For this review, take the finished solid that the model builds, in its own axes (mm). A direction names the side the tool comes from. Round coordinates to 2 decimals unless told otherwise and drop trailing zeros. Write each loop counter-clockwise with the first axis right and the second up, starting at its lowest first coordinate (ties: lowest second). Pieces come first, ordered by that corner, then holes. Notation, with made-up numbers: (88, 82) - (118, 82) arc R9 ccw to (118, 86) - close; hole circle Ø10 at (63.25, -40). An arc over 180 degrees is marked (long way). Answer in a Markdown table with one row per item. Add a question column.
from build123d import *

# Parameters (mm, degrees)
SKETCH1_R                 = 21
BOSS_EXTRUDE1_DEPTH       = 2
SKETCH2_R                 = 20
BOSS_EXTRUDE2_DEPTH       = 74
SKETCH3_R                 = 12.5
CUT_EXTRUDE1_DEPTH        = 77
SKETCH4_W                 = 8
SKETCH4_H                 = 7
CUT_EXTRUDE2_DEPTH        = 76
M6X1_0_TAPPED_HOLE1_D     = 5
M6X1_0_TAPPED_HOLE1_DEPTH = 8.497848452
M6X1_0_TAPPED_HOLE1_TIP   = 1.502151548


with BuildPart() as part:
    # Sketch1 → Boss-Extrude1 (new body)
    with BuildSketch(Plane.XY):
        Circle(SKETCH1_R)
    extrude(amount=BOSS_EXTRUDE1_DEPTH)

    # Sketch2 → Boss-Extrude2 (add)
    with BuildSketch(Plane.XY.offset(2)):
        Circle(SKETCH2_R)
    extrude(amount=BOSS_EXTRUDE2_DEPTH)

    # Sketch3 → Cut-Extrude1 (cut, through all)
    with BuildSketch(Plane(origin=(0, 0, 0), x_dir=(-1, 0, 0), z_dir=(0, 0, -1))):
        Circle(SKETCH3_R)
    extrude(amount=-CUT_EXTRUDE1_DEPTH, mode=Mode.SUBTRACT)

    # Sketch4 → Cut-Extrude2 (cut)
    with BuildSketch(Plane(origin=(0, 0, 0), x_dir=(-1, 0, 0), z_dir=(0, 0, -1))):
        with Locations((0, 12.5)):
            Rectangle(SKETCH4_W, SKETCH4_H)
    extrude(amount=-CUT_EXTRUDE2_DEPTH, mode=Mode.SUBTRACT)

    # M6x1.0 Tapped Hole1
    with Locations(Plane(origin=(0, -20, 0), x_dir=(-1, 0, 0), z_dir=(0, -1, 0))):
        with Locations((0, -56)):
            Hole(M6X1_0_TAPPED_HOLE1_D / 2, depth=M6X1_0_TAPPED_HOLE1_DEPTH)
            with Locations((0, 0, -(M6X1_0_TAPPED_HOLE1_DEPTH + M6X1_0_TAPPED_HOLE1_TIP / 2))):  # 118° drill point
                Cone(0, M6X1_0_TAPPED_HOLE1_D / 2, M6X1_0_TAPPED_HOLE1_TIP, mode=Mode.SUBTRACT)


solid = part.part
Q1. Add section C-C on z = 15. State the section outline as (x, y) points.
Q2. Tool access review of faces 4 (the face through (0, 16, 37)), 5 (the face through (-4.336, -19.524, 38.482)), 6 (the face through (0, -13, 76)): name each direction out of +Z, -Z, +X, -X, +Y, -Y from which nothing blocks a thin tool from reaching the whole face with its end or side.
Q3. Add section A-A on y = -4.5. State the section outline as (x, z) points, then the cut area to 3 significant figures.
Q4. To check wall thickness, follow probe 1 along Y at (x, z) = (0, 46); probe 2 along X at (y, z) = (10.5, 4); probe 3 along Y at (x, z) = (0, 55.5). State the ranges of each line that lie inside material, in increasing order.
Q5. Insertion check: pin 1 Ø4 at (y, z) = (11.5, 49) entering from -X; pin 2 Ø1.5 at (y, z) = (-10, 50) entering from +X; pin 3 Ø1.2 at (y, z) = (14, 28.5) entering from +X. Each pin has a flat end and moves straight along its axis. Give the tip position at first contact, or say it passes through.
Q6. Add section B-B on x = 5.5. State the section outline as (y, z) points.
Q7. Add section D-D on z = 56. State the section outline as (x, y) points.
Q8. Draft analysis for pull direction Y (two halves, no side actions). For faces 1 (the face through (20.03, 6.31, 0.99)), 2 (the face through (-4, 14, 37)), 3 (the face through (-0.54, -16.07, 58.44)), state which applies: released by +Y, released by -Y, zero draft, split by the parting line, or undercut.
Answer sheet:
| question | item | result |
|---|---|---|
| 1 | outline | circle Ø40 at (0, 0); hole (-4, 11.84) arc R12.5 ccw (long way) to (4, 11.84) - (4, 16) - (-4, 16) - close |
| 2 | face 4 | +Z, -Z |
| 2 | face 5 | +Z |
| 2 | face 6 | +Z, +X, -X, +Y, -Y |
| 3 | outline | (-20.51, 0) - (-11.66, 0) - (-11.66, 76) - (-19.49, 76) - (-19.49, 2) - (-20.51, 2) - close; (11.66, 0) - (20.51, 0) - (20.51, 2) - (19.49, 2) - (19.49, 76) - (11.66, 76) - close |
| 3 | area | 1,190 mm² |
| 4 | probe 1 | y = -20 to -12.5, 16 to 20 |
| 4 | probe 2 | x = -17.02 to -6.78, 6.78 to 17.02 |
| 4 | probe 3 | y = 16 to 20 |
| 5 | pin 1 | stops at x = -17.6 |
| 5 | pin 2 | stops at x = 17.73 |
| 5 | pin 3 | stops at x = 14.85 |
| 6 | outline | (-20.27, 0) - (-11.22, 0) - (-11.22, 76) - (-19.23, 76) - (-19.23, 2) - (-20.27, 2) - close; (11.22, 0) - (20.27, 0) - (20.27, 2) - (19.23, 2) - (19.23, 76) - (11.22, 76) - close |
| 7 | outline | (-4, 11.84) - (-4, 16) - (4, 16) - (4, 11.84) arc R12.5 cw to (2.5, -12.25) - (2.5, -19.84) arc R20 ccw (long way) to (-2.5, -19.84) - (-2.5, -12.25) arc R12.5 cw to start |
| 8 | face 1 | split by the parting line |
| 8 | face 2 | undercut |
| 8 | face 3 | zero draft |
